```python
from build123d import *

# Parameters (mm, degrees)
F0_W     = 10
F0_H     = 100
F1_DEPTH = 10
F2_R     = 0.25
F3_DEPTH = 10.001
F4_R     = 1
F5_DEPTH = 10.001


with BuildPart() as f1:
    # F0 (on Front) → F1 (new body)
    with BuildSketch(Plane.XZ):
        with Locations((5, 50)):
            Rectangle(F0_W, F0_H)
    extrude(amount=F1_DEPTH)

    # F2 (on face) → F3 (cut, through all)
    with BuildSketch(Plane.XZ.offset(10)):
        with Locations((0, 50)):
            Circle(F2_R)
        with Locations((0, 38)):
            Circle(F2_R)
        with Locations((0, 26)):
            Circle(F2_R)
        with Locations((0, 14)):
            Circle(F2_R)
    extrude(amount=-F3_DEPTH, mode=Mode.SUBTRACT)

    # F4 (on Front) → F5 (cut, through all)
    with BuildSketch(Plane.XZ):
        with Locations((5, 85)):
            Circle(F4_R)
        with Locations((5, 60)):
            Circle(F4_R)
        with Locations((5, 35)):
            Circle(F4_R)
        with Locations((5, 10)):
            Circle(F4_R)
    extrude(amount=F5_DEPTH, mode=Mode.SUBTRACT)


solid = f1.part
```
CAD build for the part. Positions are in the model's coordinates, mm. Coordinates: 2 decimals unless noted, no trailing zeros. Write each loop counter-clockwise with the first axis right and the second up, starting at its lowest first coordinate (ties: lowest second). Pieces come first, ordered by that corner, then holes. Notation, with made-up numbers: (79, -25) -> (84, -25) arc R11 ccw to (84, -10) -> close; hole circle Ø7 at (61, 10.25). An arc over 180 degrees is marked (long way). Use CSV: the item, a comma, the result in double quotes. Start each with the question number.
Item 1: Wall check: probe 1 along Z at (x, y) = (5, -3); probe 2 along X at (y, z) = (-4.25, 60); probe 3 along Z at (x, y) = (4.25, -3.25). Give the ranges that are in metal, low to high.
Item 2: Band-saw the part on A-A, the plane z = 85. Write the cut outline in (x, y), plus the area to 3 significant figures.
Item 3: Two-plate mould, pull along Z, no slides. Class faces 1 (the flat face through (0, -5, 44)), 2 (the flat face through (5, -5, 100)), 3 (the flat face through (5, -5, 0)), 4 (the cylindrical face through (5, -5, 36)): +Z half, -Z half, draft (parallel to the pull), parting line (faces both ways), or undercut.
Response values:
1,probe 1,"z = 0 to 9, 11 to 34, 36 to 59, 61 to 84, 86 to 100"
1,probe 2,"x = 0 to 4, 6 to 10"
1,probe 3,"z = 0 to 9.34, 10.66 to 34.34, 35.66 to 59.34, 60.66 to 84.34, 85.66 to 100"
2,outline,"(0, -10) -> (4, -10) -> (4, 0) -> (0, 0) -> close; (6, -10) -> (10, -10) -> (10, 0) -> (6, 0) -> close"
2,area,"80.0 mm2"
3,face 1,"draft"
3,face 2,"+Z half"
3,face 3,"-Z half"
3,face 4,"undercut"
